The listing builds one solid part. Answer for the finished solid, in the listing's coordinates (mm). A direction names the side the tool comes from. Give positions to 0.01 mm unless a question says otherwise; leave off trailing zeros. Write each loop counter-clockwise with the first axis right and the second up, starting at its lowest first coordinate (ties: lowest second). Pieces come first, ordered by that corner, then holes.
```python
from build123d import *

# Parameters (mm, degrees)
SKETCH_R           = 8.5
SKETCH_R_2         = 1.5
PAD_DEPTH          = 2
SKETCH001_R        = 2
PAD001_DEPTH       = 6
POLARPATTERN_COUNT = 4


with BuildPart() as part:
    # Sketch → Pad (new body)
    with BuildSketch(Plane.XY):
        Circle(SKETCH_R)
        Circle(SKETCH_R_2, mode=Mode.SUBTRACT)
    extrude(amount=PAD_DEPTH)

    # Sketch001 → Pad001 (new body)
    with BuildSketch(Plane.XY.offset(2)):
        with Locations((6, 0)):
            Circle(SKETCH001_R)
    pad001 = extrude(amount=PAD001_DEPTH)

    # PolarPattern: Pad001 ×4 about axis
    polarpattern_axis = Axis((0, 0, 2), (0, 0, 1))
    for i in range(1, POLARPATTERN_COUNT):
        add(pad001.rotate(polarpattern_axis, i * 360 / POLARPATTERN_COUNT))


solid = part.part
```
Item 1: A cutting plane is placed at A-A, the plane y = 0. Give the vertices of the cut face in (x, z), plus the area to 3 significant figures.
Conclusion:
outline: (-8.5, 0) - (-1.5, 0) - (-1.5, 2) - (-4, 2) - (-4, 8) - (-8, 8) - (-8, 2) - (-8.5, 2) - close; (1.5, 0) - (8.5, 0) - (8.5, 2) - (8, 2) - (8, 8) - (4, 8) - (4, 2) - (1.5, 2) - close
area: 76.0 mm2
Item 2: Each of these flat-tipped pins is pushed along its axis until it touches: P1, Ø1.5, axis at x = 3.5, z = 7, coming from the +Y side; P2, Ø3, axis at x = 0.5, z = 7, coming from the +Y side; P3, Ø1.5, axis at y = 6.5, z = 2, coming from the -X side. Where does it stop, or does it pass through?
Conclusion:
P1: stops at y = 0.97
P2: stops at y = 8
P3: stops at x = -6.26
Item 3: A cutting plane is placed at C-C, the plane z = 4. Give the vertices of the cut face in (x, y), plus the area to 3 significant figures.
Conclusion:
outline: circle Ø4 at (-6, 0); circle Ø4 at (0, -6); circle Ø4 at (0, 6); circle Ø4 at (6, 0)
area: 50.3 mm2
Item 4: A cutting plane is placed at D-D, the plane x = -6. Give the vertices of the cut face in (y, z), plus the area to 3 significant figures.
Conclusion:
outline: (-6.02, 0) - (6.02, 0) - (6.02, 2) - (2, 2) - (2, 8) - (-2, 8) - (-2, 2) - (-6.02, 2) - close
area: 48.1 mm2
Item 5: Which of the six approach directions +Z, -Z, +X, -X, +Y, -Y give full straight-line access (tool end or side, diameter ignored) to faces 4 (the face through (-4.4, 1.2, 5)), 5 (the face through (4.57, 7.167, 0.986))?
Conclusion:
face 4: +Z
face 5: +Z, -Z
Item 6: Determine the mould class of faces 1 (the face through (1.2, 4.4, 5)), 2 (the face through (4.4, -1.2, 5)), 3 (the face through (6, 0, 8)) for opening direction Y: pulls with the +Y half, pulls with the -Y half, needs draft (parallel to the pull), parting line crosses it, or undercut.
Conclusion:
face 1: undercut
face 2: parting line crosses it
face 3: needs draft
Item 7: Consider probe 1 along Y at (x, z) = (0, 0.5); probe 2 along Z at (x, y) = (7, -4.75); probe 3 along X at (y, z) = (-1.25, 2.75). Determine where each line is inside the solid, lowest interval first.
Conclusion:
probe 1: y = -8.5 to -1.5, 1.5 to 8.5
probe 2: z = 0 to 2
probe 3: x = -7.56 to -4.44, 4.44 to 7.56
